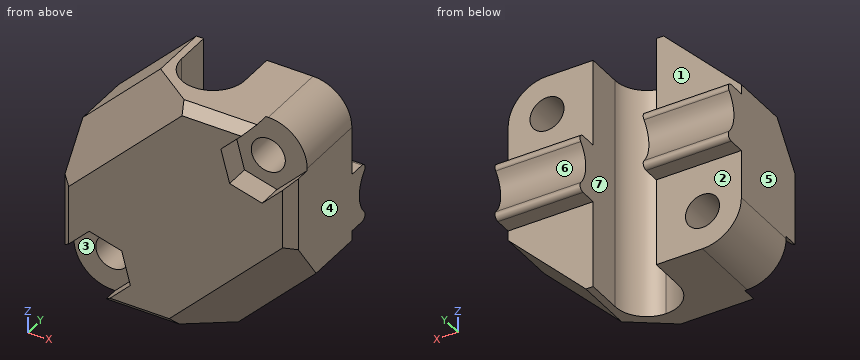
from build123d import *

# Parameters (mm, degrees)
SKETCH_1_W               = 24
SKETCH_1_H               = 24
EXTRUDE_1_DEPTH          = 10
CUT_EXTRUDE_1_DEPTH      = 29.635642127
CUT_EXTRUDE_1_DEPTH_BACK = 29.635642127
EXTRUDE_2_DEPTH          = 8.75
SKETCH_5_R               = 1.75
CUT_EXTRUDE_3_DEPTH      = 20.697715604
CHAMFER_1_SIZE           = 8
FILLET_1_R               = 4
FILLET_2_R               = 0.5
CHAMFER_2_SIZE           = 4
SKETCH_6_R               = 1.75
CUT_EXTRUDE_4_DEPTH      = 2.5
CHAMFER_3_SIZE           = 1


with BuildPart() as part:
    # 草图1 → 凸台-拉伸1 (new body)
    with BuildSketch(Plane(origin=(0, 0, 0), x_dir=(1, 0, 0), z_dir=(0, 1, 0))):
        Rectangle(SKETCH_1_W, SKETCH_1_H)
    extrude(amount=EXTRUDE_1_DEPTH)

    # 草图2 → 切除-拉伸1 (cut, two sides)
    with BuildSketch(Plane.XY.offset(12)) as cut_extrude_1_sk:
        with BuildLine():
            Line((-3.25, 10), (-3.25, 6.3))
            ThreePointArc((-3.25, 6.3), (-2.298097039, 8.598097039), (0, 9.55))
            Line((0, 9.55), (0, 10))
            Line((0, 10), (-3.25, 10))
        make_face()
        with BuildLine():
            ThreePointArc((0, 9.55), (2.298097039, 8.598097039), (3.25, 6.3))
            Line((3.25, 6.3), (3.25, 10))
            Line((3.25, 10), (0, 10))
            Line((0, 10), (0, 9.55))
        make_face()
        with BuildLine():
            ThreePointArc((-3.25, 6.3), (-2.298097039, 4.001902961), (0, 3.05))
            Line((0, 3.05), (0, 6.3))
            Line((0, 6.3), (-3.25, 6.3))
        make_face()
        with BuildLine():
            Line((0, 6.3), (0, 3.05))
            ThreePointArc((0, 3.05), (2.298097039, 4.001902961), (3.25, 6.3))
            Line((3.25, 6.3), (0, 6.3))
        make_face()
        with BuildLine():
            Line((-3.25, 6.3), (0, 6.3))
            Line((0, 6.3), (0, 9.55))
            ThreePointArc((0, 9.55), (-2.298097039, 8.598097039), (-3.25, 6.3))
        make_face()
        with BuildLine():
            Line((0, 9.55), (0, 6.3))
            Line((0, 6.3), (3.25, 6.3))
            ThreePointArc((3.25, 6.3), (2.298097039, 8.598097039), (0, 9.55))
        make_face()
    extrude(amount=CUT_EXTRUDE_1_DEPTH, mode=Mode.SUBTRACT)
    extrude(cut_extrude_1_sk.sketch, amount=-CUT_EXTRUDE_1_DEPTH_BACK, mode=Mode.SUBTRACT)

    # 草图4 → 凸台-拉伸2 (add)
    with BuildSketch(Plane(origin=(12, 0, 0), x_dir=(0, 0, -1), z_dir=(1, 0, 0))):
        with BuildLine():
            Line((-3, 10), (3, 10))
            Line((3, 10), (3, 13.25))
            ThreePointArc((3, 13.25), (0, 11.25), (-3, 13.25))
            Line((-3, 13.25), (-3, 10))
        make_face()
    extrude_2 = extrude(amount=-EXTRUDE_2_DEPTH)

    # 镜向2: 凸台-拉伸2 across plane
    add(extrude_2.mirror(Plane(origin=(0, 0, 0), x_dir=(0, 0, 1), z_dir=(1, 0, 0))))

    # 草图5 → 切除-拉伸3 (cut, through all)
    with BuildSketch(Plane(origin=(0, 10, 0), x_dir=(1, 0, 0), z_dir=(0, 1, 0))):
        with Locations(Location((-8, 8, 0), (0, 0, 270))):
            Circle(SKETCH_5_R)
        with Locations(Location((8, -8, 0), (0, 0, 90))):
            Circle(SKETCH_5_R)
    extrude(amount=-CUT_EXTRUDE_3_DEPTH, mode=Mode.SUBTRACT)

    # 倒角1
    chamfer_1_edges = [part.edges().sort_by_distance(p)[0] for p in [
        (-12, 5, 12),
        (12, 5, -12),
    ]]
    chamfer(chamfer_1_edges, length=CHAMFER_1_SIZE)

    # 圆角1
    fillet_1_edges = [part.edges().sort_by_distance(p)[0] for p in [
        (12, 5, 12),
        (-12, 5, -12),
    ]]
    fillet(fillet_1_edges, radius=FILLET_1_R)

    # 圆角2
    fillet_2_edges = [part.edges().sort_by_distance(p)[0] for p in [
        (7.625, 13.25, 3),
        (7.625, 13.25, -3),
        (-7.625, 13.25, -3),
        (-7.625, 13.25, 3),
    ]]
    fillet(fillet_2_edges, radius=FILLET_2_R)

    # 倒角2
    chamfer_2_edges = [part.edges().sort_by_distance(p)[0] for p in [
        (-8, 0, 8),
        (8, 0, -8),
    ]]
    chamfer(chamfer_2_edges, length=CHAMFER_2_SIZE)

    # 草图6 → 切除-拉伸4 (cut)
    with BuildSketch(Plane.XZ):
        Polygon((-8.896575472, -4.653934785), (-11.346065215, -7.103424528), (-7.103424528, -11.346065215), (-4.653934785, -8.896575472), (-5.550510257, -5.550510257), align=None)
        with Locations(Location((-8, -8, 0), (0, 0, 90))):
            Circle(SKETCH_6_R, mode=Mode.SUBTRACT)
        with BuildLine():
            Line((-12, -8), (-12, -7.757359313))
            Line((-12, -7.757359313), (-18.417133027, -14.17449234))
            Line((-18.417133027, -14.17449234), (-14.17449234, -18.417133027))
            Line((-14.17449234, -18.417133027), (-7.757359313, -12))
            Line((-7.757359313, -12), (-8, -12))
            ThreePointArc((-8, -12), (-10.828427125, -10.828427125), (-12, -8))
        make_face()
        with Locations(Location((-8, -8, 0), (0, 0, 90))):
            Circle(SKETCH_6_R)
        Polygon((-11.346065215, -7.103424528), (-7.103424528, -11.346065215), (-10.449489743, -10.449489743), align=None)
        with BuildLine():
            Line((-10.449489743, -10.449489743), (-11.346065215, -7.103424528))
            Line((-11.346065215, -7.103424528), (-12, -7.757359313))
            Line((-12, -7.757359313), (-12, -8))
            ThreePointArc((-12, -8), (-10.828427125, -10.828427125), (-8, -12))
            Line((-8, -12), (-7.757359313, -12))
            Line((-7.757359313, -12), (-7.103424528, -11.346065215))
            Line((-7.103424528, -11.346065215), (-10.449489743, -10.449489743))
        make_face()
        Polygon((5.550510257, 5.550510257), (4.653934785, 8.896575472), (7.103424528, 11.346065215), (11.346065215, 7.103424528), (8.896575472, 4.653934785), align=None)
        with Locations(Location((8, 8, 0), (0, 0, 270))):
            Circle(SKETCH_6_R, mode=Mode.SUBTRACT)
        with Locations(Location((8, 8, 0), (0, 0, 270))):
            Circle(SKETCH_6_R)
        Polygon((7.103424528, 11.346065215), (10.449489743, 10.449489743), (11.346065215, 7.103424528), align=None)
        with BuildLine():
            Line((8, 12), (7.757359313, 12))
            Line((7.757359313, 12), (7.103424528, 11.346065215))
            Line((7.103424528, 11.346065215), (10.449489743, 10.449489743))
            Line((10.449489743, 10.449489743), (11.346065215, 7.103424528))
            Line((11.346065215, 7.103424528), (12, 7.757359313))
            Line((12, 7.757359313), (12, 8))
            ThreePointArc((12, 8), (10.828427125, 10.828427125), (8, 12))
        make_face()
        with BuildLine():
            Line((18.417133027, 14.17449234), (14.17449234, 18.417133027))
            Line((14.17449234, 18.417133027), (7.757359313, 12))
            Line((7.757359313, 12), (8, 12))
            ThreePointArc((8, 12), (10.828427125, 10.828427125), (12, 8))
            Line((12, 8), (12, 7.757359313))
            Line((12, 7.757359313), (18.417133027, 14.17449234))
        make_face()
    extrude(amount=-CUT_EXTRUDE_4_DEPTH, mode=Mode.SUBTRACT)

    # 倒角3
    chamfer_3_edges = [part.edges().sort_by_distance(p)[0] for p in [
        (4.707106781, 0, 12),
        (-4.707106781, 0, -12),
        (12, 0, 4.707106781),
        (-12, 0, -4.707106781),
    ]]
    chamfer(chamfer_3_edges, length=CHAMFER_3_SIZE)


solid = part.part
For this review, take the finished solid that the model builds, in its own axes (mm). Face numbers are marked on the shaded views. A direction names the side the tool comes from. Give positions to 0.01 mm unless a question says otherwise; leave off trailing zeros. Loops run counter-clockwise (first coordinate to the right, second up) from the corner with the lowest first, then second, coordinate; pieces in that order, holes last. Notation, with made-up numbers: M 65,62.5 L 83,62.5 A29 ccw 83,99.5 Z; hole C 72.5,31 d2. An arc over 180 degrees is marked long. Answer as a JSON object with one key per item and string values. Group by question number.
Q1. Add section D-D on x = -5. Give the boundary of the cut face in (y, z).
Q2. Insertion check: P1, Ø3.5, axis at x = -8.5, z = -9, coming from the -Y side; P2, Ø2, axis at x = -3.5, z = -9, coming from the +Y side; P3, Ø0.9, axis at x = -8, y = 11, coming from the +Z side; P4, Ø2, axis at x = 8, z = 8, coming from the -Y side. Each pin has a flat end and moves straight along its axis. Give the tip position at first contact, or say it passes through.
Q3. Mouldability with a two-part tool opening along X and no side actions: class the marked faces 4, 5, 6 and 7 as +X half, -X half, draft (parallel to the pull), parting line (faces both ways), or undercut.
Q4. Add section C-C on z = -10.25. Give the boundary of the cut face in (x, y).
Q5. For probe 1 along X at (y, z) = (6.75, -8); probe 2 along X at (y, z) = (9.5, -1.5); probe 3 along X at (y, z) = (6.75, -7.5), list the stretches that pass through material, from the lowest coordinate up. Write a range as [from, to].
Q6. Add section A-A on y = 9.25. Give the boundary of the cut face in (x, z).
Q7. Add section B-B on y = 5.75. Give the boundary of the cut face in (x, z).
Q8. Tool access review of the marked faces 1, 2 and 3: name each direction out of +Z, -Z, +X, -X, +Y, -Y from which nothing blocks a thin tool from reaching the whole face with its end or side.
Checked values:
{
 "1": {"outline": "M 0,-11 L 1,-12 L 10,-12 L 10,-3 L 11.7,-3 A0.5 ccw 12.08,-2.17 A3.25 cw 12.08,2.17 A0.5 ccw 11.7,3 L 10,3 L 10,11 L 4,11 L 0,5.34 L 0,-7.61 L 2.5,-7.61 L 2.5,-9.24 L 0,-9.24 Z"},
 "2": {"P1": "y = 2.5", "P2": "y = 10", "P3": "z = 3", "P4": "through"},
 "3": {"face 4": "+X half", "face 5": "-X half", "face 6": "draft", "face 7": "undercut"},
 "4": {"outline": "M -11.31,2.5 L -6.01,2.5 L -6.01,0 L 0.09,0 L 5.75,4 L 5.75,10 L 3.25,10 L 3.25,6.3 A3.25 cw -3.25,6.3 L -3.25,10 L -11.31,10 Z"},
 "5": {"probe 1": "[-12, -9.75], [-6.25, -3.25], [3.25, 8]", "probe 2": "[-12, -3.25], [3.25, 12]", "probe 3": "[-12, -9.68], [-6.32, -3.25], [3.25, 8.5]"},
 "6": {"outline": "M -12,-8 A4 ccw -8,-12 L -3.25,-12 L -3.25,12 L -4,12 L -12,4 Z; M 3.25,-12 L 4,-12 L 12,-4 L 12,8 A4 ccw 8,12 L 3.25,12 Z; hole C -8,-8 d3.5; hole C 8,8 d3.5"},
 "7": {"outline": "M -12,-8 A4 ccw -8,-12 L -3.2,-12 L -3.2,12 L -4,12 L -12,4 Z; M 3.2,-12 L 4,-12 L 12,-4 L 12,8 A4 ccw 8,12 L 3.2,12 Z; hole C -8,-8 d3.5; hole C 8,8 d3.5"},
 "8": {"face 1": "+Z, +X, -X, +Y", "face 2": "-Z, +X, -X, +Y", "face 3": "-Y"}
}
